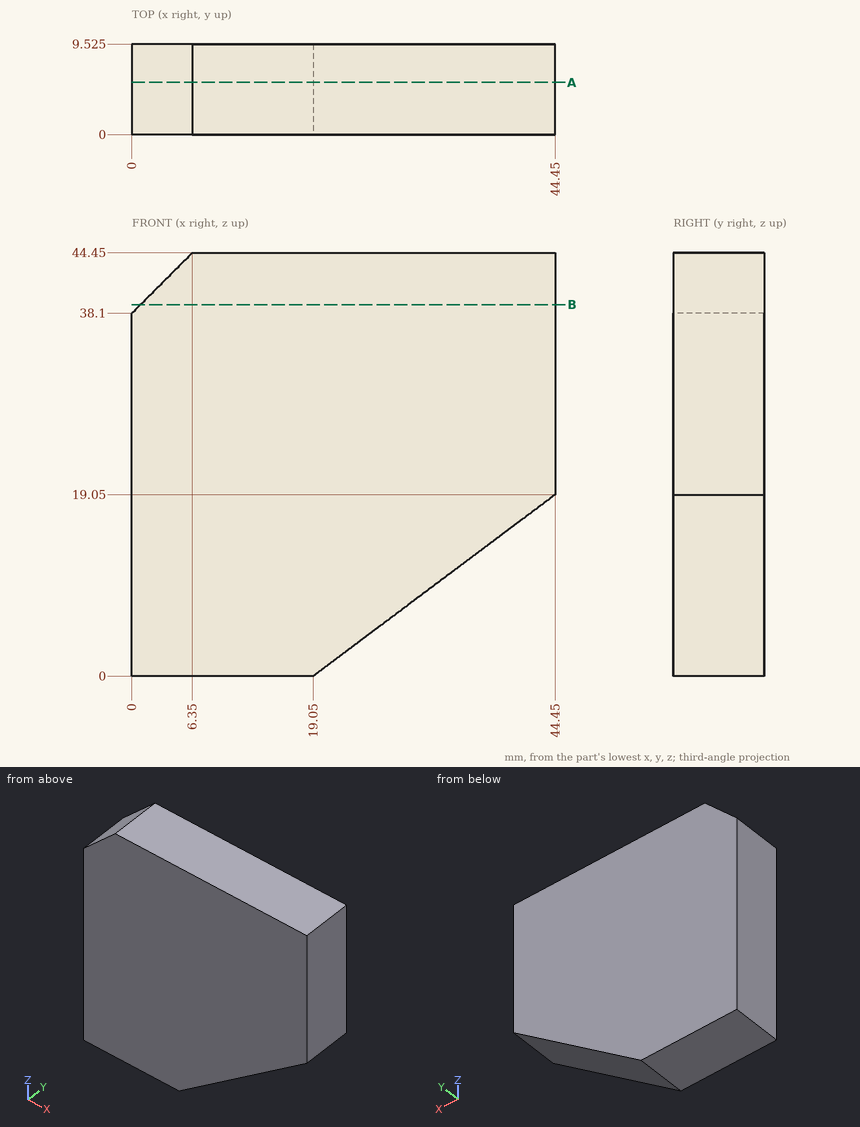
Can you work these out from the drawing? Everything is in mm from the part's minimum corner. Give positions to 0.01 mm unless a question says otherwise; leave off trailing zeros. Order: outer loops, then holes, each group sorted by start corner. A loop starts at its lowest first (then second) coordinate and runs counter-clockwise, first axis right, second up. Notation, with made-up numbers: M -7,0 L 50,0 A14 ccw 50,25 Z; hole C -9.5,82 d10. An arc over 180 degrees is marked long. Use a Markdown table: item, result. Add a question column.
1. Suppose I cut it at A-A (y = 5.5). List the corners of the cut face in (x, z) for me.
2. I need wall thicknesses on probe 1 along X at (y, z) = (5.5, 5.5); probe 2 along Z at (x, y) = (33.5, 8.75); probe 3 along Z at (x, y) = (40, 7.5). Which ranges of each line are inside material? Lowest first, please. Write a range as from..to.
3. Suppose I cut it at B-B (z = 39). List the corners of the cut face in (x, y) for me (3 decimals), and give its area (3 significant figures).
Results list:
| question | item | result |
|---|---|---|
| 1 | outline | M 0,0 L 19.05,0 L 44.45,19.05 L 44.45,44.45 L 6.35,44.45 L 0,38.1 Z |
| 2 | probe 1 | x = 0..26.38 |
| 2 | probe 2 | z = 10.84..44.45 |
| 2 | probe 3 | z = 15.71..44.45 |
| 3 | outline | M 0.9,0 L 44.45,0 L 44.45,9.525 L 0.9,9.525 Z |
| 3 | area | 415 mm² |
